Answer from the drawing. Dimensions are ordinates in mm from the lowest x, y and z of the part. Coordinates: 2 decimals unless noted, no trailing zeros. Write each loop counter-clockwise with the first axis right and the second up, starting at its lowest first coordinate (ties: lowest second). Pieces come first, ordered by that corner, then holes. Notation, with made-up numbers: (28.5, -33.75) -> (63.5, -33.75) arc R31 ccw to (63.5, -6.75) -> close; hole circle Ø11 at (47, -39.75). An arc over 180 degrees is marked (long way). Answer as a JSON object with one key per item and string values. Group by question number.
(1) Find section D-D (z = 4). Give the vertices of the cut face in (x, y), then the cut area to 3 significant figures.
(2) Find section B-B (z = 16.5). Give the vertices of the cut face in (x, y), then the cut area to 3 significant figures.
(3) Find section C-C (z = 22.5). Give the vertices of the cut face in (x, y), then the cut area to 3 significant figures.
(4) Find section A-A (x = 16.5). Give the vertices of the cut face in (y, z).
(5) Flat-ended cylindrical pins translate along their axes: P1, Ø1, axis at y = 2, z = 22, coming from the -X side; P2, Ø0.9, axis at y = 1.36, z = 16.5, coming from the +X side. Find the tip coordinate at first contact, or state that the pin passes through.
(6) For a pull along Z with two mould halves and no side action, classify the marked faces 1 and 2 as +Z half, -Z half, draft (parallel to the pull), parting line (faces both ways), or undercut.
(7) Straight lines are drawn through the part: L1, parallel to Z at x = 16.5, y = 1.6; L2, parallel to Z at x = 16.5, y = 0.8; L3, parallel to X at y = 2.1, z = 26.5. For each, find the intervals that lie inside material, in ascending order.
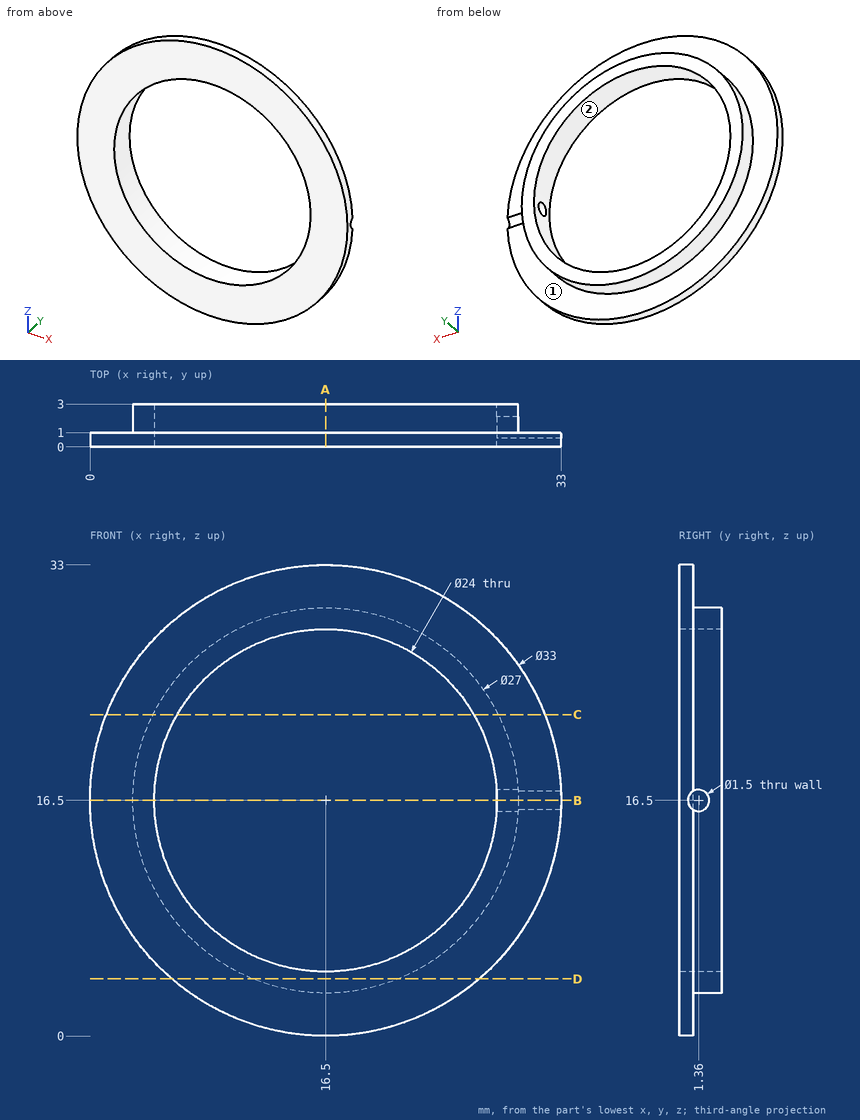
Results below:
{
 "1": {"outline": "(5.73, 0) -> (27.27, 0) -> (27.27, 1) -> (21.6, 1) -> (21.6, 3) -> (11.4, 3) -> (11.4, 1) -> (5.73, 1) -> close", "area": "41.9 mm2"},
 "2": {"outline": "(0, 0) -> (4.5, 0) -> (4.5, 3) -> (3, 3) -> (3, 1) -> (0, 1) -> close; (28.5, 0) -> (33, 0) -> (33, 0.61) -> (28.5, 0.61) -> close; (28.5, 2.11) -> (30, 2.11) -> (30, 3) -> (28.5, 3) -> close", "area": "11.6 mm2"},
 "3": {"outline": "(1.13, 0) -> (6.11, 0) -> (6.11, 3) -> (4.41, 3) -> (4.41, 1) -> (1.13, 1) -> close; (26.89, 0) -> (31.87, 0) -> (31.87, 1) -> (28.59, 1) -> (28.59, 3) -> (26.89, 3) -> close", "area": "16.8 mm2"},
 "4": {"outline": "(0, 0) -> (1, 0) -> (1, 3) -> (3, 3) -> (3, 4.5) -> (0, 4.5) -> close; (0, 28.5) -> (3, 28.5) -> (3, 30) -> (1, 30) -> (1, 33) -> (0, 33) -> close"},
 "5": {"P1": "stops at x = 3.96", "P2": "stops at x = 4.51"},
 "6": {"face 1": "draft", "face 2": "undercut"},
 "7": {"L1": "z = 3 to 4.5, 28.5 to 30", "L2": "z = 0 to 4.5, 28.5 to 33", "L3": "x = 7.43 to 9.87, 23.13 to 25.57"}
}
